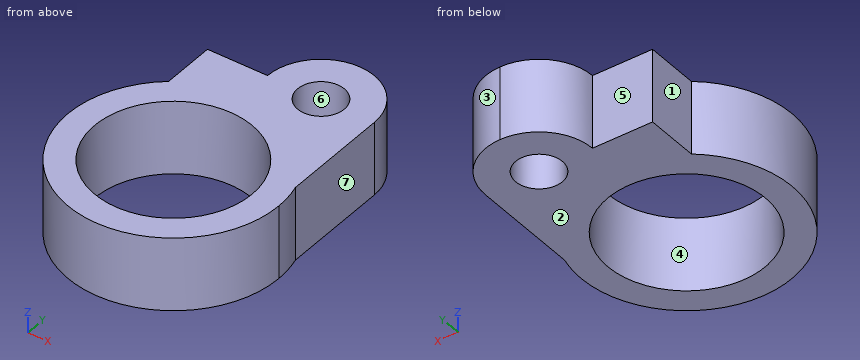
from build123d import *

# Parameters (mm, degrees)
F0_R     = 1.75
F0_R_2   = 5.9
F1_DEPTH = 5.5
F2_R     = 3.99999


# Not quite as in the source:
# - a fillet or chamfer is up to 0.001 mm smaller than in the source, because OpenCascade refuses the exact size


with BuildPart() as f1:
    # F0 (on Top) → F1 (new body)
    with BuildSketch(Plane.XY):
        with BuildLine():
            ThreePointArc((-4.881075218, 6.2116909708), (2.4746829154, 7.5023959152), (7.618924782, 2.0885366088))
            Line((7.618924782, 2.0885366088), (7.618924782, 14.2116909708))
            Line((7.618924782, 14.2116909708), (-0.381075218, 14.2116909708))
            Line((-0.381075218, 14.2116909708), (-0.381075218, 10.2116909708))
            Line((-0.381075218, 10.2116909708), (-4.881075218, 10.2116909708))
            Line((-4.881075218, 10.2116909708), (-4.881075218, 6.2116909708))
        make_face()
        with Locations((3.618924782, 10.2116909708)):
            Circle(F0_R, mode=Mode.SUBTRACT)
        with BuildLine():
            ThreePointArc((-4.881075218, 6.2116909708), (-3.4532235504, -7.1052971163), (7.9, 0))
            ThreePointArc((7.9, 0), (7.8294158715, 1.0536826425), (7.618924782, 2.0885366088))
            ThreePointArc((7.618924782, 2.0885366088), (2.4746829154, 7.5023959152), (-4.881075218, 6.2116909708))
        make_face()
        Circle(F0_R_2, mode=Mode.SUBTRACT)
    extrude(amount=F1_DEPTH)

    # F2 (radius 4 in the source; OpenCascade refuses exactly that, so slightly less here)
    f2_edges = [f1.edges().sort_by_distance(p)[0] for p in [
        (-0.381075, 14.211691, 2.75),
        (7.618925, 14.211691, 2.75),
    ]]
    fillet(f2_edges, radius=F2_R)


solid = f1.part
Verification items for the finished model (mm, model axes). Face numbers are marked on the shaded views. A direction names the side the tool comes from. Coordinates: 2 decimals unless noted, no trailing zeros. Loops run counter-clockwise (first coordinate to the right, second up) from the corner with the lowest first, then second, coordinate; pieces in that order, holes last. Notation, with made-up numbers: (84, 4.25) -> (117, 4.25) arc R27 cw to (117, 38.25) -> close; hole circle Ø11 at (66, -4). An arc over 180 degrees is marked (long way). Answer as a JSON object with one key per item and string values. Group by question number.
Item 1: Sectioned sample at A-A on x = 0. Record the boundary of the cut face in (y, z), plus the area to 3 significant figures.
Item 2: Depth check by flat-ended pin: pin 1 (1.3 mm diameter, centred on x = -3.5, z = 1.5, fed in from +Y); pin 2 (3 mm diameter, centred on x = 5, z = 4, fed in from -Y). Enter the tip coordinate at first touch or a pass-through.
Item 3: Scan lines: probe 1 along Y at (x, z) = (2.5, 1.9); probe 2 along Y at (x, z) = (3.75, 1.3); probe 3 along Y at (x, z) = (-2.25, 2.75). Record each from-to range of solid material in increasing order.
Item 4: Sectioned sample at D-D on x = 4.25. Record the boundary of the cut face in (y, z).
Item 5: Tool access check on the marked faces 5, 6 and 7. Record the directions out of +Z, -Z, +X, -X, +Y, -Y that give a thin tool (end or side, any length) a straight path to the whole face; none if there is none.
Item 6: Sectioned sample at B-B on y = 9. Record the boundary of the cut face in (x, z).
Item 7: Sectioned sample at C-C on z = 0.5. State how many separate pieces and enclosed holes the cut face has, plus the area to 3 significant figures.
Item 8: Mould release check, pull along X, two halves, no side actions. Record for the marked faces 1, 2, 3 and 4: +X half, -X half, draft (parallel to the pull), parting line (faces both ways), or undercut.
Evaluation:
{
 "1": {"outline": "(-7.9, 0) -> (-5.9, 0) -> (-5.9, 5.5) -> (-7.9, 5.5) -> close; (5.9, 0) -> (11.92, 0) -> (11.92, 5.5) -> (5.9, 5.5) -> close", "area": "44.1 mm²"},
 "2": {"pin 1": "stops at y = 10.21", "pin 2": "stops at y = -7.08"},
 "3": {"probe 1": "y = -7.49 to -5.34, 5.34 to 8.87, 11.56 to 14.05", "probe 2": "y = -6.95 to -4.55, 4.55 to 8.47, 11.96 to 14.21", "probe 3": "y = -7.57 to -5.45, 5.45 to 10.21"},
 "4": {"outline": "(-6.66, 0) -> (-4.09, 0) -> (-4.09, 5.5) -> (-6.66, 5.5) -> close; (4.09, 0) -> (8.58, 0) -> (8.58, 5.5) -> (4.09, 5.5) -> close; (11.84, 0) -> (14.16, 0) -> (14.16, 5.5) -> (11.84, 5.5) -> close"},
 "5": {"face 5": "+Z, -Z, -X, +Y", "face 6": "+Z, -Z", "face 7": "+Z, -Z, +X, +Y"},
 "6": {"outline": "(-4.88, 0) -> (2.36, 0) -> (2.36, 5.5) -> (-4.88, 5.5) -> close; (4.88, 0) -> (7.62, 0) -> (7.62, 5.5) -> (4.88, 5.5) -> close"},
 "7": {"separate pieces": "1", "enclosed holes": "2", "area": "145 mm²"},
 "8": {"face 1": "-X half", "face 2": "draft", "face 3": "+X half", "face 4": "undercut"}
}
